```python
from build123d import *

# Parameters (mm, degrees)
SKETCH_W      = 187
SKETCH_H      = 66
SKETCH_R      = 4
SKETCH_R_2    = 3
SKETCH_R_3    = 3.5
SKETCH_R_4    = 9
SKETCH_R_5    = 1.75
SKETCH_W_2    = 73
SKETCH_H_2    = 27
SKETCH_W_3    = 45.5
SKETCH_H_3    = 14
PAD_DEPTH     = 2
SKETCH001_R   = 2.75
SKETCH001_R_2 = 1.25
SKETCH001_R_3 = 2.5
SKETCH001_R_4 = 3
SKETCH001_R_5 = 1.5
PAD001_DEPTH  = 9


with BuildPart() as part:
    # Sketch → Pad (new body)
    with BuildSketch(Plane.XY):
        Rectangle(SKETCH_W, SKETCH_H)
        with Locations((69.5, -16)):
            Circle(SKETCH_R, mode=Mode.SUBTRACT)
        with Locations((-12.5, -7)):
            Circle(SKETCH_R, mode=Mode.SUBTRACT)
        with Locations((-12.5, 18)):
            Circle(SKETCH_R_2, mode=Mode.SUBTRACT)
        with Locations((-48.5, -11)):
            Circle(SKETCH_R_3, mode=Mode.SUBTRACT)
        with Locations((-35.5, -11)):
            Circle(SKETCH_R_3, mode=Mode.SUBTRACT)
        with Locations((-68.5, -11)):
            Circle(SKETCH_R_4, mode=Mode.SUBTRACT)
        with Locations((-76.454951, -3.045049)):
            Circle(SKETCH_R_5, mode=Mode.SUBTRACT)
        with Locations((-60.545049, -18.954951)):
            Circle(SKETCH_R_5, mode=Mode.SUBTRACT)
        with Locations((18.5, -16)):
            Circle(SKETCH_R_3, mode=Mode.SUBTRACT)
        with Locations((38.5, -16)):
            Circle(SKETCH_R_3, mode=Mode.SUBTRACT)
        with Locations((45, 7.5)):
            Rectangle(SKETCH_W_2, SKETCH_H_2, mode=Mode.SUBTRACT)
        with Locations((-56, 14)):
            Rectangle(SKETCH_W_3, SKETCH_H_3, mode=Mode.SUBTRACT)
    extrude(amount=PAD_DEPTH)

    # Sketch001 → Pad001 (join)
    with BuildSketch(Plane.XY):
        with Locations((82.5, 23.5)):
            Circle(SKETCH001_R)
        with Locations((82.5, 23.5)):
            Circle(SKETCH001_R_2, mode=Mode.SUBTRACT)
        with Locations((7.5, 23.5)):
            Circle(SKETCH001_R)
        with Locations((7.5, 23.5)):
            Circle(SKETCH001_R_2, mode=Mode.SUBTRACT)
        with Locations((82.5, -7.5)):
            Circle(SKETCH001_R_3)
        with Locations((82.5, -7.5)):
            Circle(SKETCH001_R_2, mode=Mode.SUBTRACT)
        with Locations((7.5, -7.5)):
            Circle(SKETCH001_R_3)
        with Locations((7.5, -7.5)):
            Circle(SKETCH001_R_2, mode=Mode.SUBTRACT)
        with Locations((-22, 26.75)):
            Circle(SKETCH001_R_4)
        with Locations((-22, 26.75)):
            Circle(SKETCH001_R_5, mode=Mode.SUBTRACT)
        with Locations((-22, -26.75)):
            Circle(SKETCH001_R_4)
        with Locations((-22, -26.75)):
            Circle(SKETCH001_R_5, mode=Mode.SUBTRACT)
        with Locations((88, -26.75)):
            Circle(SKETCH001_R_4)
        with Locations((88, -26.75)):
            Circle(SKETCH001_R_5, mode=Mode.SUBTRACT)
        with Locations((88, 26.750001)):
            Circle(SKETCH001_R_4)
        with Locations((88, 26.750001)):
            Circle(SKETCH001_R_5, mode=Mode.SUBTRACT)
    extrude(amount=-PAD001_DEPTH)


solid = part.part
```
Here's how the part is built. I have some questions about the finished solid (model axes, mm). A direction names the side the tool comes from. Coordinates: 2 decimals unless noted, no trailing zeros. Order: outer loops, then holes, each group sorted by start corner. A loop starts at its lowest first (then second) coordinate and runs counter-clockwise, first axis right, second up.
1) I need wall thicknesses on line 1 (X direction, y = 13.5, z = 0.75); line 2 (Y direction, x = -22, z = -6.75); line 3 (Y direction, x = 7.5, z = -3.75). Which ranges of each line are inside material? Lowest first, please.
2) Imagine slicing it at D-D on x = -68.5. List the corners of the cut face in (y, z) for me, and give its area (3 significant figures).
3) Will these pins go through, and if not, where does the flat tip stop? pin 1 (11 mm diameter, centred on x = 38.5, y = -16, fed in from -Z); pin 2 (5.5 mm diameter, centred on x = -12.5, y = 18, fed in from -Z); pin 3 (5 mm diameter, centred on x = -22.5, z = -3, fed in from -Y).
4) Imagine slicing it at A-A on x = -35.5. List the corners of the cut face in (y, z) for me, and give its area (3 significant figures).
5) Imagine slicing it at C-C on z = -3.75. State how many separate pieces and enclosed holes the cut face has, and give its area (3 significant figures).
6) We'd pull the mould along X, two halves only. Please class faces 3 (the face through (6, -8, -9)), 4 (the face through (-22.195, -25.263, -4.437)): +X half, -X half, draft (parallel to the pull), parting line (faces both ways), or undercut.
7) Imagine slicing it at B-B on y = 5. List the corners of the cut face in (x, z) for me.
8) Which directions (+Z, -Z, +X, -X, +Y, -Y) give clear straight access to the entire face, cutting with the end or side of a thin tool? Please do faces 1 (the face through (-74.786, -2.519, 0.986)), 2 (the face through (-22, -27, 0)).
Response values:
1. line 1: x = -93.5 to -78.75, -33.25 to 8.5, 81.5 to 93.5
1. line 2: y = -29.75 to -28.25, -25.25 to -23.75, 23.75 to 25.25, 28.25 to 29.75
1. line 3: y = -10 to -8.75, -6.25 to -5, 20.75 to 22.25, 24.75 to 26.25
2. outline: (-33, 0) - (-20, 0) - (-20, 2) - (-33, 2) - close; (-2, 0) - (7, 0) - (7, 2) - (-2, 2) - close; (21, 0) - (33, 0) - (33, 2) - (21, 2) - close
2. area: 68.0 mm2
3. pin 1: stops at z = 0
3. pin 2: passes through
3. pin 3: stops at y = -29.75
4. outline: (-33, 0) - (-14.5, 0) - (-14.5, 2) - (-33, 2) - close; (-7.5, 0) - (7, 0) - (7, 2) - (-7.5, 2) - close; (21, 0) - (33, 0) - (33, 2) - (21, 2) - close
4. area: 90.0 mm2
5. separate pieces: 8
5. enclosed holes: 8
5. area: 152 mm2
6. face 3: draft
6. face 4: undercut
7. outline: (-93.5, 0) - (8.5, 0) - (8.5, 2) - (-93.5, 2) - close; (81.5, 0) - (93.5, 0) - (93.5, 2) - (81.5, 2) - close
8. face 1: +Z, -Z
8. face 2: -Z
